Here's how the part is built. I have some questions about the finished solid (model axes, mm). A direction names the side the tool comes from. Give positions to 0.01 mm unless a question says otherwise; leave off trailing zeros. Loops run counter-clockwise (first coordinate to the right, second up) from the corner with the lowest first, then second, coordinate; pieces in that order, holes last. Notation, with made-up numbers: (-7.5, -16) - (17.5, -16) arc R15 ccw to (17.5, -11) - close; hole circle Ø4 at (5.25, 55.25). An arc over 180 degrees is marked (long way). Return JSON: item names as keys, results as strings. Group by question number.
(1) If we section it at B-B (z = 13): Please give me the cut outline in (x, y).
(2) If we mould it in two halves opening along X, with no side actions, what happens to faces 1 (the flat face through (-30.5, 37, 0)), 2 (the flat face through (9, 35, 0)), 3 (the cylindrical face through (28, 37, 13))? For each: released by +X, released by -X, zero draft, split by the parting line, or undercut.
(3) If we section it at A-A (x = -25.5): Please give me the cut outline in (y, z).
(4) If we section it at C-C (y = 3): Please give me the cut outline in (x, z).
(5) I need wall thicknesses on probe 1 along X at (y, z) = (2.25, -13); probe 2 along Y at (x, z) = (-22, 3); probe 3 along Y at (x, z) = (-3, 3.5). Which ranges of each line are inside material? Lowest first, please. Write a range as [from, to].
(6) If we section it at D-D (x = 8.5): Please give me the cut outline in (y, z).
(7) On a 3-axis mill with a long thin cutter (end or side, diameter ignored), from which of +Z, -Z, +X, -X, +Y, -Y can I reach the whole of each face in a straight line? I mean faces 4 (the flat face through (-26, 35, 0)), 5 (the flat face through (-30.5, 2, 0)). Say none if no direction works.
(8) For P1, Ø3, axis at x = 25.5, z = 13, coming from the +Y side (3 decimals); P2, Ø5, axis at y = 14.5, z = -5, coming from the +X side; P3, Ø10, axis at y = 20, z = -12.5, coming from the -X side; P4, Ø3, axis at y = 24.5, z = 7.5, coming from the +X side, each with a flat end and sliding along its axis, tell me the tip position at first contact or that it passes through.
```python
from build123d import *

# Parameters (mm, degrees)
SKETCH1_W           = 61
SKETCH1_H           = 36
SKETCH1_R           = 2.5
BOSS_EXTRUDE1_DEPTH = 5
BOSS_EXTRUDE3_DEPTH = 36
SKETCH5_W           = 61
SKETCH5_H           = 36
SKETCH5_R           = 2.5
BOSS_EXTRUDE4_DEPTH = 5


with BuildPart() as part:
    # Sketch1 → Boss-Extrude1 (new body)
    with BuildSketch(Plane(origin=(0, 0, 0), x_dir=(1, 0, 0), z_dir=(0, 1, 0))):
        Rectangle(SKETCH1_W, SKETCH1_H)
        with Locations(Location((-25.5, 13, 0), (0, 0, 270))):
            Circle(SKETCH1_R, mode=Mode.SUBTRACT)
        with Locations(Location((25.5, 13, 0), (0, 0, 270))):
            Circle(SKETCH1_R, mode=Mode.SUBTRACT)
        with Locations(Location((25.5, -13, 0), (0, 0, 270))):
            Circle(SKETCH1_R, mode=Mode.SUBTRACT)
        with Locations(Location((-25.5, -13, 0), (0, 0, 270))):
            Circle(SKETCH1_R, mode=Mode.SUBTRACT)
    extrude(amount=BOSS_EXTRUDE1_DEPTH)

    # Sketch4 → Boss-Extrude3 (add)
    with BuildSketch(Plane.XY.offset(18)):
        Polygon((19.75, 5), (-11.5, 35), (-21.5, 35), (9.75, 5), align=None)
    extrude(amount=-BOSS_EXTRUDE3_DEPTH)

    # Sketch5 → Boss-Extrude4 (add)
    with BuildSketch(Plane(origin=(0, 35, 0), x_dir=(1, 0, 0), z_dir=(0, 1, 0))):
        Rectangle(SKETCH5_W, SKETCH5_H)
        with Locations(Location((-25.5, -13, 0), (0, 0, 270))):
            Circle(SKETCH5_R, mode=Mode.SUBTRACT)
        with Locations(Location((-25.5, 13, 0), (0, 0, 270))):
            Circle(SKETCH5_R, mode=Mode.SUBTRACT)
        with Locations(Location((25.5, 13, 0), (0, 0, 270))):
            Circle(SKETCH5_R, mode=Mode.SUBTRACT)
        with Locations(Location((25.5, -13, 0), (0, 0, 270))):
            Circle(SKETCH5_R, mode=Mode.SUBTRACT)
    extrude(amount=BOSS_EXTRUDE4_DEPTH)


solid = part.part
```
Values:
{
 "1": {"outline": "(-30.5, 0) - (-28, 0) - (-28, 5) - (-30.5, 5) - close; (-30.5, 35) - (-28, 35) - (-28, 40) - (-30.5, 40) - close; (-23, 0) - (23, 0) - (23, 5) - (19.75, 5) - (-11.5, 35) - (23, 35) - (23, 40) - (-23, 40) - (-23, 35) - (-21.5, 35) - (9.75, 5) - (-23, 5) - close; (28, 0) - (30.5, 0) - (30.5, 5) - (28, 5) - close; (28, 35) - (30.5, 35) - (30.5, 40) - (28, 40) - close"},
 "2": {"face 1": "released by -X", "face 2": "zero draft", "face 3": "undercut"},
 "3": {"outline": "(0, -18) - (5, -18) - (5, -15.5) - (0, -15.5) - close; (0, -10.5) - (5, -10.5) - (5, 10.5) - (0, 10.5) - close; (0, 15.5) - (5, 15.5) - (5, 18) - (0, 18) - close; (35, -18) - (40, -18) - (40, -15.5) - (35, -15.5) - close; (35, -10.5) - (40, -10.5) - (40, 10.5) - (35, 10.5) - close; (35, 15.5) - (40, 15.5) - (40, 18) - (35, 18) - close"},
 "4": {"outline": "(-30.5, -18) - (30.5, -18) - (30.5, 18) - (-30.5, 18) - close; hole circle Ø5 at (-25.5, -13); hole circle Ø5 at (-25.5, 13); hole circle Ø5 at (25.5, -13); hole circle Ø5 at (25.5, 13)"},
 "5": {"probe 1": "[-30.5, -28], [-23, 23], [28, 30.5]", "probe 2": "[0, 5], [35, 40]", "probe 3": "[0, 5], [17.24, 26.84], [35, 40]"},
 "6": {"outline": "(0, -18) - (5, -18) - (5, 18) - (0, 18) - close; (6.2, -18) - (15.8, -18) - (15.8, 18) - (6.2, 18) - close; (35, -18) - (40, -18) - (40, 18) - (35, 18) - close"},
 "7": {"face 4": "+Z, -Z, -X", "face 5": "+Z, -Z, -X, +Y, -Y"},
 "8": {"P1": "through", "P2": "x = 12.46", "P3": "x = -11.08", "P4": "x = 1"}
}
